```python
from build123d import *

# Parameters (mm, degrees)
F0_R      = 1.8579854111
F1_DEPTH  = 25
F2_DEPTH  = 25
F3_R      = 11.5448753259
F4_DEPTH  = 80
F5_DEPTH  = 3
F6_DEPTH  = 3
F7_R      = 5.3876087587
F8_DEPTH  = 25.001
F9_DEPTH  = 3
F10_DEPTH = 1
F11_DEPTH = 3


with BuildPart() as f1:
    # F0 (on Front) → F1 (new body)
    with BuildSketch(Plane.XZ):
        with BuildLine():
            ThreePointArc((19.3358495207, -8.192980124), (20.5797575294, -4.1801411498), (21, 0))
            ThreePointArc((21, 0), (16.2024401229, 13.3596756721), (4.0018158033, 20.6151757275))
            ThreePointArc((4.0018158033, 20.6151757275), (0.7235399919, 20.987531772), (-2.5725958403, 20.8418269507))
            ThreePointArc((-2.5725958403, 20.8418269507), (-17.8139656813, 11.1203698997), (-19.8541737852, -6.8419137168))
            ThreePointArc((-19.8541737852, -6.8419137168), (-18.5375056732, -9.8671618723), (-16.7632536804, -12.6488468267))
            ThreePointArc((-16.7632536804, -12.6488468267), (-0.7235399919, -20.987531772), (15.8523579818, -13.7732620107))
            ThreePointArc((15.8523579818, -13.7732620107), (17.8139656813, -11.1203698997), (19.3358495207, -8.192980124))
        make_face()
        with BuildLine():
            ThreePointArc((-2.5725958403, 20.8418269507), (0.7235399919, 20.987531772), (4.0018158033, 20.6151757275))
            Line((4.0018158033, 20.6151757275), (4.0018158033, 30.1565360278))
            ThreePointArc((4.0018158033, 30.1565360278), (0.7146099815, 33.4437418496), (-2.5725958403, 30.1565360278))
            Line((-2.5725958403, 30.1565360278), (-2.5725958403, 20.8418269507))
        make_face()
        with Locations((0.7146099815, 30.1565360278)):
            Circle(F0_R, mode=Mode.SUBTRACT)
        with BuildLine():
            ThreePointArc((-16.7632536804, -12.6488468267), (-18.5375056732, -9.8671618723), (-19.8541737852, -6.8419137168))
            Line((-19.8541737852, -6.8419137168), (-28.1172341919, -11.6125938669))
            ThreePointArc((-28.1172341919, -11.6125938669), (-29.3204350301, -16.103000527), (-24.83002837, -17.3062013653))
            Line((-24.83002837, -17.3062013653), (-16.7632536804, -12.6488468267))
        make_face()
        with Locations((-26.473631281, -14.4593976161)):
            Circle(F0_R, mode=Mode.SUBTRACT)
        with BuildLine():
            Line((27.4026242104, -12.8503346625), (19.3358495207, -8.192980124))
            ThreePointArc((19.3358495207, -8.192980124), (17.8139656813, -11.1203698997), (15.8523579818, -13.7732620107))
            Line((15.8523579818, -13.7732620107), (24.1154183885, -18.5439421609))
            ThreePointArc((24.1154183885, -18.5439421609), (28.6058250486, -17.3407413226), (27.4026242104, -12.8503346625))
        make_face()
        with Locations((25.7590212994, -15.6971384117)):
            Circle(F0_R, mode=Mode.SUBTRACT)
    extrude(amount=F1_DEPTH)

    # F2 (add): faces of the model
    f2_faces = [f1.faces().sort_by_distance(p)[0] for p in [
        (0, 0, 0),
        (0, -25, 0),
    ]]
    extrude(f2_faces, amount=F2_DEPTH, dir=(0, 1, 0))

    # F3 (on Front) → F4 (join)
    with BuildSketch(Plane.XZ):
        Circle(F3_R)
    extrude(amount=F4_DEPTH)

    # F5 (add): faces of the model
    f5_faces = [f1.faces().sort_by_distance(p)[0] for p in [
        (0, -80, 0),
        (-1.771197573, -25, 25.4991814892),
    ]]
    extrude(f5_faces, amount=F5_DEPTH)

    # F6 (add): a face of the model
    f6_faces = [f1.faces().sort_by_distance(p)[0] for p in [
        (-1.771197573, -28, 25.4991814892),
    ]]
    extrude(f6_faces, amount=F6_DEPTH)

    # F7 (on Front) → F8 (cut, through all)
    with BuildSketch(Plane.XZ):
        Circle(F7_R)
    extrude(amount=-F8_DEPTH, mode=Mode.SUBTRACT)

    # F9 (add): a face of the model
    f9_faces = [f1.faces().sort_by_distance(p)[0] for p in [
        (-1.771197573, -31, 25.4991814892),
    ]]
    extrude(f9_faces, amount=F9_DEPTH)

    # F10 (add): a face of the model
    f10_faces = [f1.faces().sort_by_distance(p)[0] for p in [
        (-1.771197573, -34, 25.4991814892),
    ]]
    extrude(f10_faces, amount=F10_DEPTH)

    # F11 (add): a face of the model
    f11_faces = [f1.faces().sort_by_distance(p)[0] for p in [
        (0, -83, 0),
    ]]
    extrude(f11_faces, amount=F11_DEPTH)


solid = f1.part
```
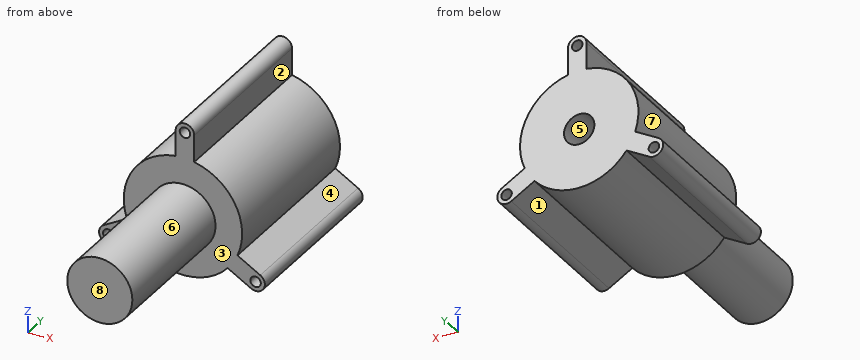
Geometry check sheet. Reference: the model listing, model coordinates, mm. Face numbers are marked on the shaded views. A direction names the side the tool comes from. Coordinates: 2 decimals unless noted, no trailing zeros. Loops run counter-clockwise (first coordinate to the right, second up) from the corner with the lowest first, then second, coordinate; pieces in that order, holes last. Notation, with made-up numbers: (36.5, 23.25) - (81.5, 23.25) arc R24 cw to (81.5, 41.25) - close; hole circle Ø8 at (-1.5, 16). An arc over 180 degrees is marked (long way). One line per item, written item: value. Start each with the question number.
(1) Cross-section at D-D on y = -22. Enter the section's corners in (x, z), plus the area to 3 significant figures.
(2) Mould release check, pull along Z, two halves, no side actions. Record for the marked faces 6, 7 and 8: released by +Z, released by -Z, zero draft, split by the parting line, or undercut.
(3) Material ranges on line 1 (Z direction, x = 0, y = 11); line 2 (X direction, y = -26.5, z = 24.5); line 3 (Z direction, x = -3, y = 13), recorded low to high. Write a range as [from, to].
(4) Cross-section at B-B on x = 0. Enter the section's corners in (y, z), plus the area to 3 significant figures.
(5) Depth check by flat-ended pin: P1, Ø12, axis at x = -14, z = 13.5, coming from the -Y side; P2, Ø5, axis at y = -4.5, z = 27, coming from the +X side; P3, Ø6.5, axis at x = 0, z = 0, coming from the +Y side. Enter the tip coordinate at first touch or a pass-through.
(6) Cross-section at C-C on y = 2. Enter the section's corners in (x, z).
(7) Tool access check on the marked faces 1, 2, 3, 4 and 5. Record the directions out of +Z, -Z, +X, -X, +Y, -Y that give a thin tool (end or side, any length) a straight path to the whole face; none if there is none.
(8) Cross-section at A-A on z = 0. Enter the section's corners in (x, y).
Results below:
1. outline: (-28.12, -11.61) arc R3.29 ccw to (-24.83, -17.31) - (-16.76, -12.65) arc R21 ccw to (15.85, -13.77) - (24.12, -18.54) arc R3.29 ccw to (27.4, -12.85) - (19.34, -8.19) arc R21 ccw to (4, 20.62) - (4, 30.16) arc R3.29 ccw to (-2.57, 30.16) - (-2.57, 20.84) arc R21 ccw to (-19.85, -6.84) - close; hole circle Ø3.72 at (-26.47, -14.46); hole circle Ø3.72 at (0.71, 30.16); hole circle Ø3.72 at (25.76, -15.7)
1. area: 1,590 mm2
2. face 6: split by the parting line
2. face 7: undercut
2. face 8: zero draft
3. line 1: z = [-21, -5.39], [5.39, 28.44], [31.87, 33.37]
3. line 2: x = [-2.57, 4]
3. line 3: z = [-20.78, -4.48], [4.48, 20.78]
4. outline: (-86, -11.54) - (-35, -11.54) - (-35, -21) - (25, -21) - (25, -5.39) - (0, -5.39) - (0, 5.39) - (25, 5.39) - (25, 28.44) - (-35, 28.44) - (-35, 11.54) - (-86, 11.54) - close; (-35, 31.87) - (25, 31.87) - (25, 33.37) - (-35, 33.37) - close
4. area: 3,960 mm2
5. P1: stops at y = -35
5. P2: stops at x = 4
5. P3: stops at y = 0
6. outline: (-28.12, -11.61) arc R3.29 ccw to (-24.83, -17.31) - (-16.76, -12.65) arc R21 ccw to (15.85, -13.77) - (24.12, -18.54) arc R3.29 ccw to (27.4, -12.85) - (19.34, -8.19) arc R21 ccw to (4, 20.62) - (4, 30.16) arc R3.29 ccw to (-2.57, 30.16) - (-2.57, 20.84) arc R21 ccw to (-19.85, -6.84) - close; hole circle Ø3.72 at (-26.47, -14.46); hole circle Ø10.78 at (0, 0); hole circle Ø3.72 at (0.71, 30.16); hole circle Ø3.72 at (25.76, -15.7)
7. face 1: -Z, +Y, -Y
7. face 2: +Z, +X, +Y, -Y
7. face 3: -Y
7. face 4: +X, +Y, -Y
7. face 5: +Y
8. outline: (-21, -35) - (-11.54, -35) - (-11.54, -86) - (11.54, -86) - (11.54, -35) - (21, -35) - (21, 25) - (5.39, 25) - (5.39, 0) - (-5.39, 0) - (-5.39, 25) - (-21, 25) - close
